from build123d import *

# Parameters (mm, degrees)
SKETCH1_W           = 176.143624501
SKETCH1_H           = 20.199458611
SKETCH1_R           = 5.3975
SKETCH1_R_2         = 2.73924182
BOSS_EXTRUDE1_DEPTH = 6.858
SKETCH5_W           = 310.671331162
SKETCH5_H           = 20.199458611
BOSS_EXTRUDE4_DEPTH = 5.334


with BuildPart() as part:
    # Sketch1 → Boss-Extrude1 (new body)
    with BuildSketch(Plane.ZY):
        with Locations((220.759467441, -42.412189395)):
            Rectangle(SKETCH1_W, SKETCH1_H)
        with Locations((145.296375125, -42.412189394)):
            Circle(SKETCH1_R, mode=Mode.SUBTRACT)
        with Locations((184.665923862, -42.412189394)):
            Circle(SKETCH1_R_2, mode=Mode.SUBTRACT)
    boss_extrude1 = extrude(amount=BOSS_EXTRUDE1_DEPTH)

    # Sketch5 → Boss-Extrude4 (add)
    with BuildSketch(Plane.XY.offset(308.831279691)):
        with Locations((148.477665581, -42.412189395)):
            Rectangle(SKETCH5_W, SKETCH5_H)
    extrude(amount=BOSS_EXTRUDE4_DEPTH)

    # Mirror1: Boss-Extrude1 across plane
    add(boss_extrude1.mirror(Plane.ZY.offset(-148.477665581)))


solid = part.part
Check sheet for the modelled part. Datum: model origin and axes. Units: mm. A direction names the side the tool comes from. Round coordinates to 2 decimals unless told otherwise and drop trailing zeros. Order: outer loops, then holes, each group sorted by start corner. A loop starts at its lowest first (then second) coordinate and runs counter-clockwise, first axis right, second up.
(1) Scan lines: probe 1 along X at (y, z) = (-43.75, 230); probe 2 along Z at (x, y) = (181.5, -48.5). Record each from-to range of solid material in increasing order.
(2) Cross-section at B-B, the plane z = 146. Enter the section's corners in (x, y).
(3) Cross-section at A-A, the plane z = 248.5. Enter the section's corners in (x, y), and give its area (3 significant figures).
(4) Draft check along Z on faces 3 (the flat face through (296.955, -42, 220)), 4 (the cylindrical face through (-3.38, -41.59, 187.28)), 5 (the flat face through (146, -42, 308.831)). Enter one of: pulls with the +Z half, pulls with the -Z half, needs draft (parallel to the pull), parting line crosses it, or undercut.
(5) Cross-section at C-C, the plane x = 231. Enter the section's corners in (y, z), and give its area (3 significant figures).
(6) Access from +Z, -Z, +X, -X, +Y, -Y to the whole of each face (thin tool, end or side, straight path). Record for faces 1 (the flat face through (0, -42, 220)), 2 (the cylindrical face through (-3.381, -42.175, 139.904)).
(7) Go/stop test with flat-tipped pins: P1, Ø9.5, axis at y = -42.41, z = 145.3, coming from the +X side; P2, Ø6, axis at x = 172.5, y = -46, coming from the -Z side; P3, Ø9, axis at y = -42.41, z = 184.67, coming from the -X side. Record where each tip stops, or that it passes through.
Check sheet entries:
1. probe 1: x = -6.86 to 0, 296.96 to 303.81
1. probe 2: z = 308.83 to 314.17
2. outline: (-6.86, -52.51) - (0, -52.51) - (0, -47.76) - (-6.86, -47.76) - close; (-6.86, -37.06) - (0, -37.06) - (0, -32.31) - (-6.86, -32.31) - close; (296.96, -52.51) - (303.81, -52.51) - (303.81, -47.76) - (296.96, -47.76) - close; (296.96, -37.06) - (303.81, -37.06) - (303.81, -32.31) - (296.96, -32.31) - close
3. outline: (-6.86, -52.51) - (0, -52.51) - (0, -32.31) - (-6.86, -32.31) - close; (296.96, -52.51) - (303.81, -52.51) - (303.81, -32.31) - (296.96, -32.31) - close
3. area: 277 mm2
4. face 3: needs draft
4. face 4: undercut
4. face 5: pulls with the -Z half
5. outline: (-52.51, 308.83) - (-32.31, 308.83) - (-32.31, 314.17) - (-52.51, 314.17) - close
5. area: 108 mm2
6. face 1: -Z, +Y, -Y
6. face 2: +X, -X
7. P1: passes through
7. P2: stops at z = 308.83
7. P3: stops at x = -6.86
